The listing builds one solid part. Answer for the finished solid, in the listing's coordinates (mm). A direction names the side the tool comes from. Give positions to 0.01 mm unless a question says otherwise; leave off trailing zeros. Return JSON: item names as keys, results as strings.
from build123d import *


with BuildPart() as f1:
    # F0 (on Right) → F1 (revolve)
    with BuildSketch(Plane.YZ):
        with BuildLine():
            Line((3, 63), (3, 51.2))
            Line((3, 51.2), (8.5, 51.2))
            Line((8.5, 51.2), (12.672783, 49.755051))
            ThreePointArc((12.672783, 49.755051), (13, 49.7), (13.327217, 49.755051))
            Line((13.327217, 49.755051), (17.5, 51.2))
            Line((17.5, 51.2), (42.255857, 51.2))
            Line((42.255857, 51.2), (42.255857, 68))
            Line((42.255857, 68), (40.255857, 68))
            Line((40.255857, 68), (35.888214, 56))
            Line((35.888214, 56), (34.638214, 56))
            Line((34.638214, 56), (30.270571, 68))
            Line((30.270571, 68), (28.970571, 68))
            Line((28.970571, 68), (28.970571, 75))
            Line((28.970571, 75), (25.970571, 75))
            Line((25.970571, 75), (21.602928, 63))
            Line((21.602928, 63), (20.352928, 63))
            Line((20.352928, 63), (15.985286, 75))
            Line((15.985286, 75), (12.985286, 75))
            Line((12.985286, 75), (8.617643, 63))
            Line((8.617643, 63), (7.367643, 63))
            Line((7.367643, 63), (3, 75))
            Line((3, 75), (0, 75))
            Line((0, 75), (0, 63))
            Line((0, 63), (3, 63))
        make_face()
    revolve(axis=Axis((0, 21.127928, 0), (0, 1, 0)))


solid = f1.part
Item 1: Which of the six approach directions +Z, -Z, +X, -X, +Y, -Y give full straight-line access (tool end or side, diameter ignored) to faces 1 (the flat face through (61, 0, -17)), 2 (the cylindrical face through (62.464, 7.984, -8.201)), 3 (the cylindrical face through (74.362, 14.464, -9.764)), 4 (the cylindrical face through (57.338, 29.611, 36.556)), 5 (the flat face through (52, 3, 0))?
Geometry results:
{"face 1": "+Z, -Z, +X, -X, -Y", "face 2": "none", "face 3": "+Y, -Y", "face 4": "+Y", "face 5": "-Y"}
Item 2: Determine the mould class of faces 6 (the flat face through (51, 42.256, -10)), 7 (the cylindrical face through (62.464, 1.521, -8.201)), 8 (the cylindrical face through (-31.154, 30.051, -40.631)), 9 (the cylindrical face through (74.362, 1.479, -9.764)) for opening direction X: +X half, -X half, draft (parallel to the pull), parting line (faces both ways), or undercut.
Geometry results:
{"face 6": "draft", "face 7": "undercut", "face 8": "undercut", "face 9": "parting line"}
Item 3: Find the intervals of material crossed by line 1 (Y direction, x = 65, z = -1.5); line 2 (Y direction, x = 42.5, z = 57); line 3 (Y direction, x = -38.5, z = 60.5), in increasing order.
Geometry results:
{"line 1": "y = 0 to 6.63, 9.35 to 19.62, 22.34 to 31.36, 39.17 to 42.26", "line 2": "y = 0 to 4.42, 11.57 to 17.4, 24.55 to 28.97", "line 3": "y = 0 to 4.2, 11.79 to 17.18, 24.77 to 28.97"}
Item 4: Given pin 1 Ø8 at (y, z) = (13, 33) entering from -X; pin 2 Ø5 at (y, z) = (28, 20) entering from -X; pin 3 Ø2 at (y, z) = (29, -47.5) entering from -X, each flat-ended and moving along its own axis, determine where each tip first touches the part or whether it passes through.
Geometry results:
{"pin 1": "stops at x = -69.17", "pin 2": "stops at x = -72.93", "pin 3": "stops at x = -58.84"}
